```python
from build123d import *

# Parameters (mm, degrees)
SKETCH1_W           = 25.4
SKETCH1_H           = 50.8
SKETCH1_W_2         = 19.05
SKETCH1_H_2         = 44.45
BOSS_EXTRUDE1_DEPTH = 762
CUT_EXTRUDE1_REACH  = 764.846
SKETCH4_R           = 14.224
SKETCH5_R           = 2.0955
CUT_EXTRUDE2_DEPTH  = 3.175
CUT_EXTRUDE3_REACH  = 764.846
SKETCH7_R           = 2.0955


with BuildPart() as part:
    # Sketch1 → Boss-Extrude1 (new body)
    with BuildSketch(Plane.XY):
        Rectangle(SKETCH1_W, SKETCH1_H)
        Rectangle(SKETCH1_W_2, SKETCH1_H_2, mode=Mode.SUBTRACT)
    extrude(amount=BOSS_EXTRUDE1_DEPTH)

    # Cut-Extrude1: up to this face of the body (flat: up to its plane)
    cut_extrude1_end = Plane(part.part.faces().sort_by_distance((-12.7, 0, 381))[0])
    # Sketch4 → Cut-Extrude1 (cut, up to the picked face)
    with BuildSketch(Plane(origin=(12.7, 0, 0), x_dir=(0, 0, -1), z_dir=(1, 0, 0)), mode=Mode.PRIVATE) as cut_extrude1_sk1:
        with Locations(Location((-190.549048411, 0, 0), (0, 0, 90))):
            Circle(SKETCH4_R)
    cut_extrude1_tool1 = split(extrude(cut_extrude1_sk1.sketch, amount=-CUT_EXTRUDE1_REACH, mode=Mode.PRIVATE), bisect_by=cut_extrude1_end, keep=Keep.BOTH, mode=Mode.PRIVATE)
    # Sketch4 → Cut-Extrude1 (cut, up to the picked face)
    with BuildSketch(Plane(origin=(12.7, 0, 0), x_dir=(0, 0, -1), z_dir=(1, 0, 0)), mode=Mode.PRIVATE) as cut_extrude1_sk2:
        with BuildLine():
            Line((-703.248048411, 14.224), (-690.548048411, 14.224))
            ThreePointArc((-690.548048411, 14.224), (-676.324048411, 0), (-690.548048411, -14.224))
            Line((-690.548048411, -14.224), (-703.248048411, -14.224))
            ThreePointArc((-703.248048411, -14.224), (-717.472048411, 0), (-703.248048411, 14.224))
        make_face()
    cut_extrude1_tool2 = split(extrude(cut_extrude1_sk2.sketch, amount=-CUT_EXTRUDE1_REACH, mode=Mode.PRIVATE), bisect_by=cut_extrude1_end, keep=Keep.BOTH, mode=Mode.PRIVATE)
    add(cut_extrude1_tool1.solids().sort_by(Axis((12.7, 0, 190.549048), (-1, 0, 0)))[0], mode=Mode.SUBTRACT)
    add(cut_extrude1_tool2.solids().sort_by(Axis((12.7, 0, 696.898048), (-1, 0, 0)))[0], mode=Mode.SUBTRACT)

    # Sketch5 → Cut-Extrude2 (cut)
    with BuildSketch(Plane.XZ.offset(25.4)):
        with Locations(Location((2.54, 264.16, 0), (0, 0, 270))):
            Circle(SKETCH5_R)
        with Locations(Location((2.54, 289.56, 0), (0, 0, 270))):
            Circle(SKETCH5_R)
        with Locations(Location((2.54, 314.96, 0), (0, 0, 270))):
            Circle(SKETCH5_R)
        with Locations(Location((-2.54, 264.16, 0), (0, 0, 180))):
            Circle(SKETCH5_R)
        with Locations(Location((-2.54, 289.56, 0), (0, 0, 180))):
            Circle(SKETCH5_R)
        with Locations(Location((-2.54, 314.96, 0), (0, 0, 180))):
            Circle(SKETCH5_R)
    extrude(amount=-CUT_EXTRUDE2_DEPTH, mode=Mode.SUBTRACT)

    # Cut-Extrude3: up to this face of the body (flat: up to its plane)
    cut_extrude3_end = Plane(part.part.faces().sort_by_distance((-12.7, 0, 375.771255471))[0])
    # Sketch7 → Cut-Extrude3 (cut, up to the picked face)
    with BuildSketch(Plane(origin=(12.7, 0, 0), x_dir=(0, 0, -1), z_dir=(1, 0, 0)), mode=Mode.PRIVATE) as cut_extrude3_sk1:
        with Locations(Location((-259.08, -15.24, 0), (0, 0, 90))):
            Circle(SKETCH7_R)
    cut_extrude3_tool1 = split(extrude(cut_extrude3_sk1.sketch, amount=-CUT_EXTRUDE3_REACH, mode=Mode.PRIVATE), bisect_by=cut_extrude3_end, keep=Keep.BOTH, mode=Mode.PRIVATE)
    # Sketch7 → Cut-Extrude3 (cut, up to the picked face)
    with BuildSketch(Plane(origin=(12.7, 0, 0), x_dir=(0, 0, -1), z_dir=(1, 0, 0)), mode=Mode.PRIVATE) as cut_extrude3_sk2:
        with Locations(Location((-284.48, -15.24, 0), (0, 0, 90))):
            Circle(SKETCH7_R)
    cut_extrude3_tool2 = split(extrude(cut_extrude3_sk2.sketch, amount=-CUT_EXTRUDE3_REACH, mode=Mode.PRIVATE), bisect_by=cut_extrude3_end, keep=Keep.BOTH, mode=Mode.PRIVATE)
    # Sketch7 → Cut-Extrude3 (cut, up to the picked face)
    with BuildSketch(Plane(origin=(12.7, 0, 0), x_dir=(0, 0, -1), z_dir=(1, 0, 0)), mode=Mode.PRIVATE) as cut_extrude3_sk3:
        with Locations(Location((-309.88, -15.24, 0), (0, 0, 90))):
            Circle(SKETCH7_R)
    cut_extrude3_tool3 = split(extrude(cut_extrude3_sk3.sketch, amount=-CUT_EXTRUDE3_REACH, mode=Mode.PRIVATE), bisect_by=cut_extrude3_end, keep=Keep.BOTH, mode=Mode.PRIVATE)
    # Sketch7 → Cut-Extrude3 (cut, up to the picked face)
    with BuildSketch(Plane(origin=(12.7, 0, 0), x_dir=(0, 0, -1), z_dir=(1, 0, 0)), mode=Mode.PRIVATE) as cut_extrude3_sk4:
        with Locations(Location((-87.63, -15.24, 0), (0, 0, 90))):
            Circle(SKETCH7_R)
    cut_extrude3_tool4 = split(extrude(cut_extrude3_sk4.sketch, amount=-CUT_EXTRUDE3_REACH, mode=Mode.PRIVATE), bisect_by=cut_extrude3_end, keep=Keep.BOTH, mode=Mode.PRIVATE)
    # Sketch7 → Cut-Extrude3 (cut, up to the picked face)
    with BuildSketch(Plane(origin=(12.7, 0, 0), x_dir=(0, 0, -1), z_dir=(1, 0, 0)), mode=Mode.PRIVATE) as cut_extrude3_sk5:
        with Locations(Location((-62.23, -15.24, 0), (0, 0, 90))):
            Circle(SKETCH7_R)
    cut_extrude3_tool5 = split(extrude(cut_extrude3_sk5.sketch, amount=-CUT_EXTRUDE3_REACH, mode=Mode.PRIVATE), bisect_by=cut_extrude3_end, keep=Keep.BOTH, mode=Mode.PRIVATE)
    # Sketch7 → Cut-Extrude3 (cut, up to the picked face)
    with BuildSketch(Plane(origin=(12.7, 0, 0), x_dir=(0, 0, -1), z_dir=(1, 0, 0)), mode=Mode.PRIVATE) as cut_extrude3_sk6:
        with Locations(Location((-113.03, -15.24, 0), (0, 0, 90))):
            Circle(SKETCH7_R)
    cut_extrude3_tool6 = split(extrude(cut_extrude3_sk6.sketch, amount=-CUT_EXTRUDE3_REACH, mode=Mode.PRIVATE), bisect_by=cut_extrude3_end, keep=Keep.BOTH, mode=Mode.PRIVATE)
    add(cut_extrude3_tool1.solids().sort_by(Axis((12.7, -15.24, 259.08), (-1, 0, 0)))[0], mode=Mode.SUBTRACT)
    add(cut_extrude3_tool2.solids().sort_by(Axis((12.7, -15.24, 284.48), (-1, 0, 0)))[0], mode=Mode.SUBTRACT)
    add(cut_extrude3_tool3.solids().sort_by(Axis((12.7, -15.24, 309.88), (-1, 0, 0)))[0], mode=Mode.SUBTRACT)
    add(cut_extrude3_tool4.solids().sort_by(Axis((12.7, -15.24, 87.63), (-1, 0, 0)))[0], mode=Mode.SUBTRACT)
    add(cut_extrude3_tool5.solids().sort_by(Axis((12.7, -15.24, 62.23), (-1, 0, 0)))[0], mode=Mode.SUBTRACT)
    add(cut_extrude3_tool6.solids().sort_by(Axis((12.7, -15.24, 113.03), (-1, 0, 0)))[0], mode=Mode.SUBTRACT)


solid = part.part
```
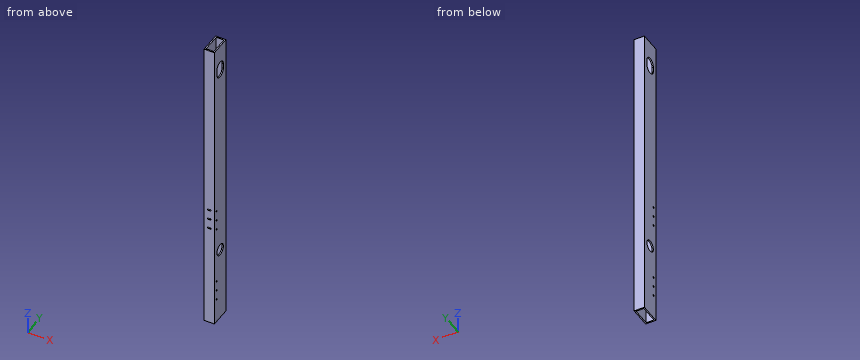
Input: part model. Units: mm. Frame: model coordinates. Round coordinates to 2 decimals unless told otherwise and drop trailing zeros. Loops run counter-clockwise (first coordinate to the right, second up) from the corner with the lowest first, then second, coordinate; pieces in that order, holes last.
1) Section query A-A on z = 422.5. Return the cut outline in (x, y) (3 decimals), plus the area to 3 significant figures.
Ans:
outline: (-12.7, -25.4) - (12.7, -25.4) - (12.7, 25.4) - (-12.7, 25.4) - close; hole (-9.525, -22.225) - (9.525, -22.225) - (9.525, 22.225) - (-9.525, 22.225) - close
area: 444 mm2
2) Pin query (flat end, axial travel): pin 1 (2.5 mm diameter, centred on y = -15.24, z = 284.48, fed in from +X); pin 2 (3.5 mm diameter, centred on x = -2.54, z = 264.16, fed in from -Y) (3 decimals). Return the tip coordinate at first contact, or that it passes through.
Ans:
pin 1: passes through
pin 2: stops at y = 22.225
3) Material intervals for line 1 (X direction, y = -23, z = 264); line 2 (X direction, y = 18, z = 407) (3 decimals); line 3 (Y direction, x = 6.5, z = 161.5) (3 decimals), sorted ascending.
Ans:
line 1: x = -12.7 to -4.63, -0.45 to 0.45, 4.63 to 12.7
line 2: x = -12.7 to -9.525, 9.525 to 12.7
line 3: y = -25.4 to -22.225, 22.225 to 25.4
4) Section query B-B on y = 3. Return the cut outline in (x, z) (3 decimals), plus the area to 3 significant figures.
Ans:
outline: (-12.7, 0) - (-9.525, 0) - (-9.525, 176.645) - (-12.7, 176.645) - close; (-12.7, 204.453) - (-9.525, 204.453) - (-9.525, 676.644) - (-12.7, 676.644) - close; (-12.7, 717.152) - (-9.525, 717.152) - (-9.525, 762) - (-12.7, 762) - close; (9.525, 0) - (12.7, 0) - (12.7, 176.645) - (9.525, 176.645) - close; (9.525, 204.453) - (12.7, 204.453) - (12.7, 676.644) - (9.525, 676.644) - close; (9.525, 717.152) - (12.7, 717.152) - (12.7, 762) - (9.525, 762) - close
area: 4,400 mm2
